```python
from build123d import *

# Parameters (mm, degrees)
SKETCH1_W           = 20
SKETCH1_H           = 58.42
SKETCH1_R           = 2.05
BOSS_EXTRUDE1_DEPTH = 7.9375
SKETCH2_R           = 4.05
CUT_EXTRUDE1_DEPTH  = 15
CHAMFER1_SIZE       = 2.48


with BuildPart() as part:
    # Sketch1 → Boss-Extrude1 (new body)
    with BuildSketch(Plane(origin=(0, -110.068674648, 0), x_dir=(1, 0, 0), z_dir=(0, 1, 0))):
        with Locations((78.333864278, -62.627324848)):
            Rectangle(SKETCH1_W, SKETCH1_H)
        with Locations(Location((78.333864278, -76.837324848, 0), (0, 0, 270))):
            Circle(SKETCH1_R, mode=Mode.SUBTRACT)
        with Locations(Location((78.333864278, -48.417324848, 0), (0, 0, 270))):
            Circle(SKETCH1_R, mode=Mode.SUBTRACT)
    extrude(amount=BOSS_EXTRUDE1_DEPTH)

    # Sketch2 → Cut-Extrude1 (cut)
    with BuildSketch(Plane(origin=(88.333864278, -1.5875, 4.936331956), x_dir=(0, 0, -1), z_dir=(1, 0, 0))):
        with Locations((-57.690992892, -108.481174648)):
            Circle(SKETCH2_R)
    extrude(amount=-CUT_EXTRUDE1_DEPTH, mode=Mode.SUBTRACT)

    # Chamfer1
    chamfer1_edges = [part.edges().sort_by_distance(p)[0] for p in [
        (78.333864278, -102.131174648, 74.787324848),
        (78.333864278, -102.131174648, 46.367324848),
    ]]
    chamfer(chamfer1_edges, length=CHAMFER1_SIZE)


solid = part.part
```
Geometry: final body of the model. Coordinates: model frame, mm. A direction names the side the tool comes from. Give positions to 0.01 mm unless a question says otherwise; leave off trailing zeros. Order: outer loops, then holes, each group sorted by start corner. A loop starts at its lowest first (then second) coordinate and runs counter-clockwise, first axis right, second up. Notation, with made-up numbers: M 84.25,83.5 L 127.25,83.5 A22 cw 127.25,103.5 Z; hole C 63,-28 d11. An arc over 180 degrees is marked long. Answer as CSV lines item,"result". Start each with the question number.
1) Cut plane B-B (y = -107). Output: boundary loops of the cut face in (x, z), then the cut area to 3 significant figures.
2) Cut plane A-A (x = 86.5). Output: boundary loops of the cut face in (y, z).
3) Line query: line 1 (Z direction, x = 78.5, y = -104.25); line 2 (Z direction, x = 85.5, y = -109); line 3 (Z direction, x = 73.75, y = -108). Output: solid intervals per line, ascending. Write a range as from..to.
4) Set-up query: faces 1 (the flat face through (72, -110.069, 62)), 2 (the cylindrical face through (80.94, -106.02, 62.54)). Return all of +Z, -Z, +X, -X, +Y, -Y with unobstructed straight access to the full face (end or side cutting, diameter ignored); none if empty.
5) First-contact query: P1, Ø4.5, axis at x = 78.33, z = 48.42, coming from the +Y side; P2, Ø3, axis at y = -108.5, z = 61, coming from the +X side. Flat tips, straight axial feed; report the tip coordinate or a pass-through.
6) Cut plane C-C (z = 62). Output: boundary loops of the cut face in (x, y).
7) Mould query, pull axis Z, two halves, no side actions, for faces 3 (the flat face through (78, -106, 33.417)), 4 (the flat face through (73.334, -108, 63)), 5 (the flat face through (78, -106, 91.837)), 6 (the conical face through (79.801, -104.491, 75.238)). Classes: +Z half, -Z half, draft (parallel to the pull), parting line (faces both ways), or undercut.
8) Cut plane D-D (y = -103.5). Output: boundary loops of the cut face in (x, z), then the cut area to 3 significant figures.
Findings below:
1,outline,"M 68.33,33.42 L 88.33,33.42 L 88.33,59.98 L 73.33,59.98 L 73.33,65.27 L 88.33,65.27 L 88.33,91.84 L 68.33,91.84 Z; hole C 78.33,48.42 d4.1; hole C 78.33,76.84 d4.1"
1,area,"1,060 mm²"
2,outline,"M -110.07,33.42 L -102.13,33.42 L -102.13,91.84 L -110.07,91.84 L -110.07,66.68 A4.05 cw -110.07,58.58 Z"
3,line 1,"z = 33.42..46.01, 50.82..74.43, 79.24..91.84"
3,line 2,"z = 33.42..58.72, 66.53..91.84"
3,line 3,"z = 33.42..59.15, 66.11..91.84"
4,face 1,"+Z, -Z, +X, -X, -Y"
4,face 2,"+X, -Y"
5,P1,"stops at y = -104.41"
5,P2,"stops at x = 73.33"
6,outline,"M 68.33,-110.07 L 73.33,-110.07 L 73.33,-106.07 L 88.33,-106.07 L 88.33,-102.13 L 68.33,-102.13 Z"
7,face 3,"-Z half"
7,face 4,"undercut"
7,face 5,"+Z half"
7,face 6,"undercut"
8,outline,"M 68.33,33.42 L 88.33,33.42 L 88.33,91.84 L 68.33,91.84 Z; hole C 78.33,48.42 d6.32; hole C 78.33,76.84 d6.32"
8,area,"1,110 mm²"
